```python
from build123d import *

# Parameters (mm, degrees)
F0_R     = 50
F1_DEPTH = 140
F2_R     = 30
F3_DEPTH = 40
F4_R     = 10
F5_DEPTH = 80


with BuildPart() as f1:
    # F0 (on Front) → F1 (new body)
    with BuildSketch(Plane.XZ):
        Circle(F0_R)
    extrude(amount=-F1_DEPTH)

    # F2 (on face) → F3 (cut)
    with BuildSketch(Plane.XZ):
        Circle(F2_R)
    extrude(amount=-F3_DEPTH, mode=Mode.SUBTRACT)

    # F4 (on face) → F5 (cut)
    with BuildSketch(Plane.XZ):
        Circle(F4_R)
    extrude(amount=-F5_DEPTH, mode=Mode.SUBTRACT)


solid = f1.part
```
The model under review builds one solid part; all positions refer to its coordinate system, in mm. A direction names the side the tool comes from. Round coordinates to 2 decimals unless told otherwise and drop trailing zeros. Order: outer loops, then holes, each group sorted by start corner. A loop starts at its lowest first (then second) coordinate and runs counter-clockwise, first axis right, second up. Notation, with made-up numbers: (-10, -14) -> (24, -14) arc R5 cw to (24, -5) -> close; hole circle Ø9 at (33, 37). An arc over 180 degrees is marked (long way). Use a Markdown table: item, result.
Q1. Tool access review of faces 5 (the flat face through (0, 80, 0)), 6 (the flat face through (22, 0, -22)): name each direction out of +Z, -Z, +X, -X, +Y, -Y from which nothing blocks a thin tool from reaching the whole face with its end or side.
Values:
| item | result |
|---|---|
| face 5 | -Y |
| face 6 | +Z, -Z, +X, -X, -Y |
Q2. We need section A-A on x = 0. Write out the cut boundary in (y, z).
Values:
| item | result |
|---|---|
| outline | (0, -50) -> (140, -50) -> (140, 50) -> (0, 50) -> (0, 30) -> (40, 30) -> (40, 10) -> (80, 10) -> (80, -10) -> (40, -10) -> (40, -30) -> (0, -30) -> close |
Q3. We need section B-B on z = 0. Write out the cut boundary in (x, y), then the cut area to 3 significant figures.
Values:
| item | result |
|---|---|
| outline | (-50, 0) -> (-30, 0) -> (-30, 40) -> (-10, 40) -> (-10, 80) -> (10, 80) -> (10, 40) -> (30, 40) -> (30, 0) -> (50, 0) -> (50, 140) -> (-50, 140) -> close |
| area | 10,800 mm^2 |
Q4. We need section C-C on y = 59.5. Write out the cut boundary in (x, z), then the cut area to 3 significant figures.
Values:
| item | result |
|---|---|
| outline | circle Ø100 at (0, 0); hole circle Ø20 at (0, 0) |
| area | 7,540 mm^2 |
Q5. We need section D-D on y = 97. Write out the cut boundary in (x, z), then the cut area to 3 significant figures.
Values:
| item | result |
|---|---|
| outline | circle Ø100 at (0, 0) |
| area | 7,850 mm^2 |
Q6. For line 1 (Z direction, x = 0, y = 65); line 2 (X direction, y = 24, z = 10); line 3 (Z direction, x = 4, y = 52), list the stretches that pass through material, from the lowest coordinate up.
Values:
| item | result |
|---|---|
| line 1 | z = -50 to -10, 10 to 50 |
| line 2 | x = -48.99 to -28.28, 28.28 to 48.99 |
| line 3 | z = -49.84 to -9.17, 9.17 to 49.84 |
Q7. Clearance check with flat-ended pins moving along their axes: P1, Ø3, axis at x = -2, y = 84, coming from the -Z side; P2, Ø5, axis at x = -33, z = -0.5, coming from the -Y side; P3, Ø4, axis at x = -37, y = 47.5, coming from the -Z side; P4, Ø1, axis at x = 0, y = 102.5, coming from the +Z side. State where each tip first meets the part, or that it passes through.
Values:
| item | result |
|---|---|
| P1 | stops at z = -50 |
| P2 | stops at y = 0 |
| P3 | stops at z = -35.71 |
| P4 | stops at z = 50 |
Q8. Mouldability with a two-part tool opening along X and no side actions: class faces 1 (the flat face through (13, 40, 0)), 2 (the cylindrical face through (-29.97, 19.72, 1.32)), 3 (the flat face through (-1, 140, 1)), 4 (the cylindrical face through (47.69, 69.02, 15.02)) as +X half, -X half, draft (parallel to the pull), parting line (faces both ways), or undercut.
Values:
| item | result |
|---|---|
| face 1 | undercut |
| face 2 | undercut |
| face 3 | draft |
| face 4 | parting line |
